Source: CAD feature listing. Evaluate the final solid. Frame: model axes, mm. Coordinates: 2 decimals unless noted, no trailing zeros. Loops run counter-clockwise (first coordinate to the right, second up) from the corner with the lowest first, then second, coordinate; pieces in that order, holes last. Notation, with made-up numbers: (76.25, 62) - (128.25, 62) arc R21 ccw to (128.25, 79) - close; hole circle Ø3 at (48.5, 57). An arc over 180 degrees is marked (long way). Write item = value, one per line. Start each with the question number.
Autodesk Inventor part; units mm, degrees
ref_plane "YZ Plane" through (0, 0, 0) normal (1, 0, 0) x (0, 1, 0)
ref_plane "XZ Plane" through (0, 0, 0) normal (0, 1, 0) x (-1, 0, 0)
ref_plane "XY Plane" through (0, 0, 0) normal (0, 0, 1) x (1, 0, 0)
sketch "CONTOURS" plane through (0, 0, 0) normal (0, 0, 1) x (1, 0, 0)
  arc A0 (28.0046, 396.7552) -> (1814.0653, 446.8716) centre (897.7889, 1250.2638) ccw
  line L0 (28.0046, 396.7552) -> (68.5769, 436.5356)
  arc A1 (91.1499, 433.6624) -> (68.5769, 436.5356) centre (78.7284, 426.182) ccw
  line L1 (91.1499, 433.6624) -> (106.0415, 408.9341)
  arc A2 (106.0415, 408.9341) -> (130.7846, 406.4993) centre (119.3197, 416.9304) ccw
  line L2 (130.7846, 406.4993) -> (251.8873, 539.6044)
  arc A3 (251.8873, 539.6044) -> (247.9235, 563.5995) centre (240.4224, 550.0355) ccw
  line L3 (247.9235, 563.5995) -> (233.1425, 571.7736)
  arc A4 (230.0082, 594.8161) -> (233.1425, 571.7736) centre (240.1597, 584.4626) ccw
  line L4 (230.0082, 594.8161) -> (269.3503, 633.3904)
  arc A5 (269.3503, 633.3904) -> (1526.2271, 633.3904) centre (897.7887, 1250.4881) ccw
  line L5 (1526.2271, 633.3904) -> (1814.0653, 446.8716)
sketch "HOLES" plane through (0, 0, 0) normal (0, 0, 1) x (1, 0, 0)
  arc A0 (288.9886, 574.6199) -> (288.8907, 580.2759) centre (286.1117, 577.3989) ccw
  line L0 (288.9886, 574.6199) -> (281.3462, 566.7082)
  arc A1 (275.6902, 566.6103) -> (281.3462, 566.7082) centre (278.4693, 569.4873) ccw
  line L1 (275.6902, 566.6103) -> (249.7976, 591.6217)
  arc A2 (249.6997, 597.2778) -> (249.7976, 591.6217) centre (252.5767, 594.4987) ccw
  line L2 (1440.2918, 203.0579) -> (1445.4546, 193.3448)
  arc A3 (1445.4546, 193.3448) -> (1450.864, 191.6901) centre (1448.9867, 195.2221) ccw
  line L3 (1450.864, 191.6901) -> (1482.6526, 208.5865)
  arc A4 (1482.6526, 208.5865) -> (1484.3073, 213.9959) centre (1480.7752, 212.1185) ccw
  line L4 (1484.3073, 213.9959) -> (1479.1445, 223.7091)
  arc A5 (1479.1445, 223.7091) -> (1473.735, 225.3638) centre (1475.6124, 221.8317) ccw
  line L5 (1473.735, 225.3638) -> (1441.9465, 208.4674)
  arc A6 (1441.9465, 208.4674) -> (1440.2918, 203.0579) centre (1443.8239, 204.9353) ccw
  line L6 (101.125, 380.1374) -> (93.4826, 372.2258)
  arc A7 (87.8266, 372.1279) -> (93.4826, 372.2258) centre (90.6056, 375.0048) ccw
  line L7 (87.8266, 372.1279) -> (61.9339, 397.1393)
  arc A8 (61.836, 402.7953) -> (61.9339, 397.1393) centre (64.713, 400.0162) ccw
  line L8 (61.836, 402.7953) -> (69.4784, 410.7069)
  arc A9 (75.1344, 410.8048) -> (69.4784, 410.7069) centre (72.3554, 407.9279) ccw
  line L9 (75.1344, 410.8048) -> (101.027, 385.7934)
  arc A10 (101.125, 380.1374) -> (101.027, 385.7934) centre (98.248, 382.9165) ccw
  line L10 (1362.2188, 382.0722) -> (1356.0415, 378.7797)
  arc A11 (1356.0415, 378.7797) -> (1354.3929, 373.3684) centre (1357.9229, 375.2498) ccw
  line L11 (1354.3929, 373.3684) -> (1411.7752, 265.7057)
  arc A12 (1411.7752, 265.7057) -> (1417.1866, 264.0571) centre (1415.3052, 267.587) ccw
  line L12 (1417.1866, 264.0571) -> (1426.8939, 269.2309)
  arc A13 (1426.8939, 269.2309) -> (1428.5424, 274.6423) centre (1425.0125, 272.7609) ccw
  line L13 (1428.5424, 274.6423) -> (1371.1601, 382.305)
  arc A14 (1371.1601, 382.305) -> (1365.7488, 383.9536) centre (1367.6302, 380.4236) ccw
  line L14 (1365.7488, 383.9536) -> (1362.2188, 382.0722)
  line L15 (249.6997, 597.2778) -> (257.3421, 605.1894)
  arc A15 (262.9981, 605.2873) -> (257.3421, 605.1894) centre (260.219, 602.4103) ccw
  line L16 (262.9981, 605.2873) -> (288.8907, 580.2759)
  line L17 (1318.5439, 432.1121) -> (1313.3811, 441.8253)
  arc A16 (1315.0357, 447.2347) -> (1313.3811, 441.8253) centre (1316.9131, 443.7027) ccw
  line L18 (1315.0357, 447.2347) -> (1346.8243, 464.1311)
  arc A17 (1352.2337, 462.4764) -> (1346.8243, 464.1311) centre (1348.7017, 460.5991) ccw
  line L19 (1352.2337, 462.4764) -> (1357.3965, 452.7633)
  arc A18 (1355.7418, 447.3538) -> (1357.3965, 452.7633) centre (1353.8645, 450.8859) ccw
  line L20 (1355.7418, 447.3538) -> (1323.9533, 430.4574)
  arc A19 (1318.5439, 432.1121) -> (1323.9533, 430.4574) centre (1322.0759, 433.9895) ccw
sketch "LETTERS" plane through (0, 0, 0) normal (0, 0, 1) x (1, 0, 0)
  line L0 (243.6817, 427.6795) -> (251.9783, 420.9747)
  line L1 (249.8017, 435.2055) -> (237.3515, 419.7995)
  line L2 (237.3515, 419.7995) -> (248.775, 410.5677)
  line L3 (261.2252, 425.9736) -> (249.8017, 435.2055)
extrude "Extrusion1" add sketch "CONTOURS" along normal blind 18
extrude "Extrusion2" cut sketch "HOLES" along normal blind 18
properties part number "Platform E4" material "Wood (Birch)"
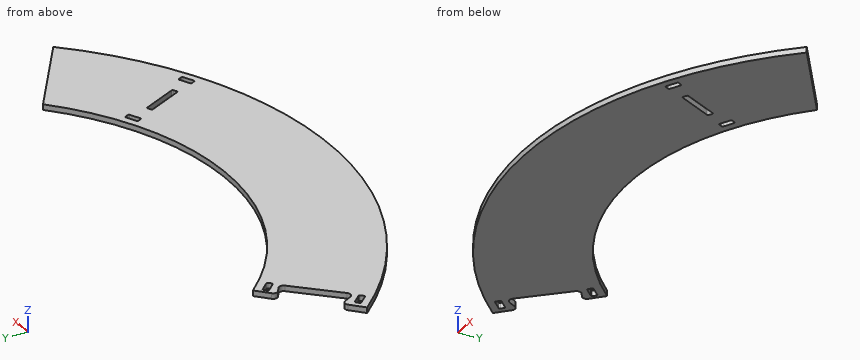
Item 1: First-contact query: pin 1 (1.5 mm diameter, centred on x = 1561.5, z = 15, fed in from +Y); pin 2 (3 mm diameter, centred on y = 188.5, z = 9.5, fed in from -X); pin 3 (1 mm diameter, centred on y = 511, z = 12, fed in from +X); pin 4 (1.5 mm diameter, centred on x = 336.5, y = 230, fed in from -Z). Flat tips, straight axial feed; report the tip coordinate or a pass-through.
Item 2: Cut plane D-D (x = 1561). Return the cut outline in (y, z), then the cut area to 3 significant figures.
Item 3: Cut plane A-A (y = 516.5). Return the cut outline in (x, z).
Item 4: Cut plane B-B (z = 7.5). State how many separate pieces and enclosed holes the cut face has, then the cut area to 3 significant figures.
Item 5: Material intervals for L1, parallel to X at y = 576, z = 12.75; L2, parallel to X at y = 544.5, z = 9.5; L3, parallel to X at y = 551.5, z = 10.25, sorted ascending. Write a range as [from, to].
Item 6: Cut plane C-C (y = 345). Return the cut outline in (x, z), then the cut area to 3 significant figures.
Responses:
q1.pin_1 = 611.02
q1.pin_2 = 297.09
q1.pin_3 = 1715.87
q1.pin_4 = 0
q2.outline = (227.94, 0) - (610.86, 0) - (610.86, 18) - (227.94, 18) - close
q2.area = 6,890 mm2
q3.outline = (230.87, 0) - (410.96, 0) - (410.96, 18) - (230.87, 18) - close; (1384.62, 0) - (1706.61, 0) - (1706.61, 18) - (1384.62, 18) - close
q4.separate_pieces = 1
q4.enclosed_holes = 5
q4.area = 558,000 mm2
q5.L1 = [228.39, 265.97], [289.86, 331.39], [1464.19, 1614.79]
q5.L2 = [254.9, 371.17], [1424.41, 1663.4]
q5.L3 = [255.85, 361.92], [1433.66, 1652.6]
q6.outline = (82.01, 0) - (1369.51, 0) - (1369.51, 18) - (82.01, 18) - close; (1391.04, 0) - (1713.57, 0) - (1713.57, 18) - (1391.04, 18) - close
q6.area = 29,000 mm2
